Source: CAD feature listing. Evaluate the final solid. Frame: model axes, mm. Face numbers are marked on the shaded views. Round coordinates to 2 decimals unless told otherwise and drop trailing zeros. Loops run counter-clockwise (first coordinate to the right, second up) from the corner with the lowest first, then second, coordinate; pieces in that order, holes last. Notation, with made-up numbers: (44.25, -38) - (79.25, -38) arc R13 ccw to (79.25, -13) - close; hole circle Ø11 at (22, 55.25). An arc over 180 degrees is marked (long way). Use CSV: the item, a comma, the result in double quotes. Start each with the question number.
from build123d import *

# Parameters (mm, degrees)
SKETCH1_R           = 1.5
BOSS_EXTRUDE1_DEPTH = 49
CHAMFER1_SIZE       = 0.5
CHAMFER1_SIZE2      = 2
CHAMFER2_SIZE       = 2
CHAMFER2_SIZE2      = 0.5
SKETCH2_W           = 6
SKETCH2_H           = 5
CUT_EXTRUDE1_DEPTH  = 0.5


with BuildPart() as part:
    # Sketch1 → Boss-Extrude1 (new body)
    with BuildSketch(Plane(origin=(0, 0, 0), x_dir=(1, 0, 0), z_dir=(0, 1, 0))):
        Circle(SKETCH1_R)
    extrude(amount=BOSS_EXTRUDE1_DEPTH)

    # Chamfer1
    chamfer1_edges = [part.edges().sort_by_distance(p)[0] for p in [
        (-1.5, 0, 0),
    ]]
    chamfer1_side = [part.faces().sort_by_distance(p)[0] for p in [
        (0, 0, 0),
    ]]
    chamfer(chamfer1_edges, length=CHAMFER1_SIZE, length2=CHAMFER1_SIZE2, reference=chamfer1_side[0])

    # Chamfer2
    chamfer2_edges = [part.edges().sort_by_distance(p)[0] for p in [
        (-1.5, 49, 0),
    ]]
    chamfer2_side = [part.faces().sort_by_distance(p)[0] for p in [
        (-1.5, 25.5, 0),
    ]]
    chamfer(chamfer2_edges, length=CHAMFER2_SIZE, length2=CHAMFER2_SIZE2, reference=chamfer2_side[0])

    # Sketch2 → Cut-Extrude1 (cut)
    with BuildSketch(Plane(origin=(1.5, 0, 0), x_dir=(0, 0, -1), z_dir=(1, 0, 0))):
        with Locations((0, 9.5)):
            Rectangle(SKETCH2_W, SKETCH2_H)
    extrude(amount=-CUT_EXTRUDE1_DEPTH, mode=Mode.SUBTRACT)


solid = part.part
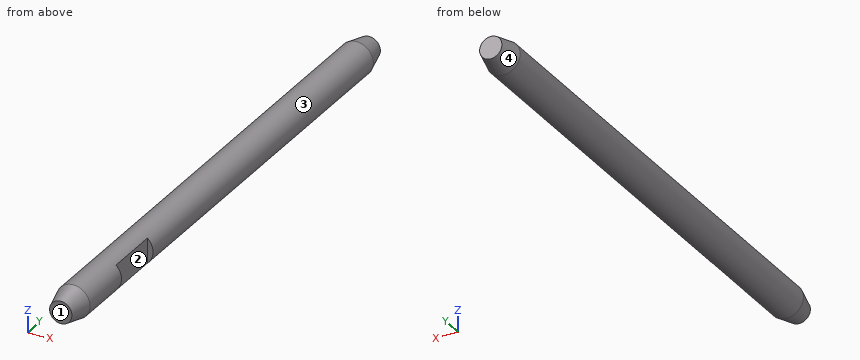
1. Section query A-A on z = 0. Return the cut outline in (x, y).
2. Line query: line 1 along X through (y, z) = (15, 1); line 2 along Z through (x, y) = (0.55, 30). Output: solid intervals per line, ascending.
3. Contact query for a flat-ended pin moving along its axis: P1, Ø1.5, axis at y = 7.5, z = 1, coming from the +X side. Output: stop coordinate, or through.
4. Mould query, pull axis Y, two halves, no side actions, for the marked faces 1, 2, 3 and 4. Classes: +Y half, -Y half, draft (parallel to the pull), parting line (faces both ways), or undercut.
5. Section query B-B on y = 28. Return the cut outline in (x, z).
Values:
1,outline,"(-1.5, 2) - (-1, 0) - (1, 0) - (1.5, 2) - (1.5, 7) - (1, 7) - (1, 12) - (1.5, 12) - (1.5, 47) - (1, 49) - (-1, 49) - (-1.5, 47) - close"
2,line 1,"x = -1.12 to 1.12"
2,line 2,"z = -1.4 to 1.4"
3,P1,"stops at x = 1.43"
4,face 1,"-Y half"
4,face 2,"undercut"
4,face 3,"draft"
4,face 4,"+Y half"
5,outline,"circle Ø3 at (0, 0)"
